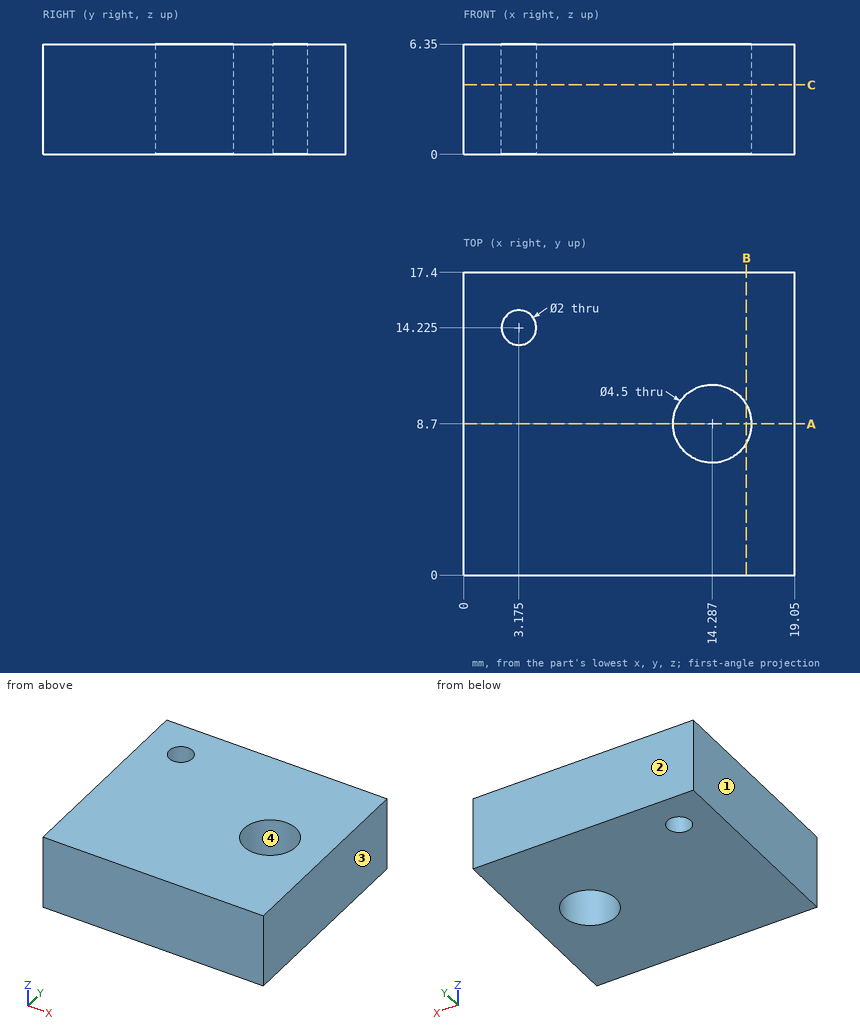
Here's the drawing with two shaded views (mm, measured from the low corner). I have some questions. Give positions to 0.01 mm unless a question says otherwise; leave off trailing zeros. Order: outer loops, then holes, each group sorted by start corner. A loop starts at its lowest first (then second) coordinate and runs counter-clockwise, first axis right, second up. Notation, with made-up numbers: (-29, 2.5) - (20, 2.5) arc R14 cw to (20, 29.5) - close; hole circle Ø9 at (-31.75, 38.25). An arc over 180 degrees is marked (long way). Write each question's results on one line, items separated by ' | '.
1) Suppose I cut it at A-A, the plane y = 8.7. Write out the boundary of the cut face in (x, z).
Final values:
outline: (0, 0) - (12.04, 0) - (12.04, 6.35) - (0, 6.35) - close; (16.54, 0) - (19.05, 0) - (19.05, 6.35) - (16.54, 6.35) - close
2) Please list where these lines run through material, in increasing order: line 1 along Y through (x, z) = (14, 3); line 2 along Y through (x, z) = (3, 2.5); line 3 along X through (y, z) = (8.5, 1.75). Write a range as [from, to].
Final values:
line 1: y = [0, 6.47], [10.93, 17.4] | line 2: y = [0, 13.24], [15.21, 17.4] | line 3: x = [0, 12.05], [16.53, 19.05]
3) Suppose I cut it at B-B, the plane x = 16.25. Write out the boundary of the cut face in (y, z).
Final values:
outline: (0, 0) - (7.6, 0) - (7.6, 6.35) - (0, 6.35) - close; (9.8, 0) - (17.4, 0) - (17.4, 6.35) - (9.8, 6.35) - close
4) Suppose I cut it at C-C, the plane z = 4. Give the number of separate pieces and of enclosed holes in the cut face.
Final values:
separate pieces: 1 | enclosed holes: 2
5) If we mould it in two halves opening along X, with no side actions, what happens to the marked faces 1, 2, 3 and 4? For each: pulls with the +X half, pulls with the -X half, needs draft (parallel to the pull), parting line crosses it, or undercut.
Final values:
face 1: pulls with the -X half | face 2: needs draft | face 3: pulls with the +X half | face 4: undercut
